Can you work these out from the model? Positions are in its coordinate system, mm. A direction names the side the tool comes from. Give positions to 0.01 mm unless a question says otherwise; leave off trailing zeros. Loops run counter-clockwise (first coordinate to the right, second up) from the corner with the lowest first, then second, coordinate; pieces in that order, holes last. Notation, with made-up numbers: M -36.5,-35 L 1.5,-35 A23 cw 1.5,-15 Z; hole C 9.5,0 d7. An arc over 180 degrees is marked long. Answer as a JSON object with one key per item and string values.
```python
from build123d import *

# Parameters (mm, degrees)
SKETCH1_W                = 32
SKETCH1_H                = 15
BOSS_EXTRUDE1_DEPTH      = 4
BOSS_EXTRUDE2_START      = 4
SKETCH1_3_W              = 32
SKETCH1_3_H              = 5
BOSS_EXTRUDE2_DEPTH      = 23.5
BOSS_EXTRUDE3_DEPTH      = 17
M3_CLEARANCE_HOLE1_D     = 3.6
M3_CLEARANCE_HOLE1_DEPTH = 10
M3_CLEARANCE_HOLE1_TIP   = 1.081549114


with BuildPart() as part:
    # Sketch1 → Boss-Extrude1 (new body)
    with BuildSketch(Plane(origin=(0, 0, 0), x_dir=(1, 0, 0), z_dir=(0, 1, 0))):
        with Locations((0, 2.5)):
            Rectangle(SKETCH1_W, SKETCH1_H)
    extrude(amount=BOSS_EXTRUDE1_DEPTH)

    # Sketch1<3> → Boss-Extrude2 (add)
    with BuildSketch(Plane(origin=(0, 0, 0), x_dir=(1, 0, 0), z_dir=(0, 1, 0)).offset(BOSS_EXTRUDE2_START)):
        with Locations((0, -2.5)):
            Rectangle(SKETCH1_3_W, SKETCH1_3_H)
    extrude(amount=BOSS_EXTRUDE2_DEPTH)

    # Sketch2 → Boss-Extrude3 (add)
    with BuildSketch(Plane.XY.offset(5)):
        Polygon((-6.5, 2), (-6.5, 25.5), (-2.5, 25.5), (-2.5, 27.5), (-9, 27.5), (-9, 0), (9, 0), (9, 27.5), (2.5, 27.5), (2.5, 25.5), (6.5, 25.5), (6.5, 2), align=None)
    extrude(amount=BOSS_EXTRUDE3_DEPTH)

    # M3 Clearance Hole1
    with Locations(Plane(origin=(0, 4, 0), x_dir=(1, 0, 0), z_dir=(0, 1, 0))):
        with Locations((-10, 5), (10, 5)):
            Hole(M3_CLEARANCE_HOLE1_D / 2, depth=M3_CLEARANCE_HOLE1_DEPTH)
            with Locations((0, 0, -(M3_CLEARANCE_HOLE1_DEPTH + M3_CLEARANCE_HOLE1_TIP / 2))):  # 118° drill point
                Cone(0, M3_CLEARANCE_HOLE1_D / 2, M3_CLEARANCE_HOLE1_TIP, mode=Mode.SUBTRACT)


solid = part.part
```
1) Suppose I cut it at D-D, the plane z = 12. Write out the boundary of the cut face in (x, y), and give its area (4 significant figures).
Answer list:
{"outline": "M -9,0 L 9,0 L 9,27.5 L 2.5,27.5 L 2.5,25.5 L 6.5,25.5 L 6.5,2 L -6.5,2 L -6.5,25.5 L -2.5,25.5 L -2.5,27.5 L -9,27.5 Z", "area": "179.5 mm^2"}
2) Please list where these lines run through material, in increasing order: line 1 along X through (y, z) = (1.25, -5); line 2 along X through (y, z) = (15.75, 8); line 3 along Z through (x, y) = (10, 0.8). Write a range as from..to.
Answer list:
{"line 1": "-16..-11.8, -8.2..8.2, 11.8..16", "line 2": "-9..-6.5, 6.5..9", "line 3": "-10..-6.8, -3.2..5"}
3) Suppose I cut it at C-C, the plane y = 23. Write out the boundary of the cut face in (x, z), and give its area (3 significant figures).
Answer list:
{"outline": "M -16,0 L 16,0 L 16,5 L 9,5 L 9,22 L 6.5,22 L 6.5,5 L -6.5,5 L -6.5,22 L -9,22 L -9,5 L -16,5 Z", "area": "245 mm^2"}
4) Will these pins go through, and if not, where does the flat tip stop? pin 1 Ø12 at (x, y) = (-6, 16) entering from +Z; pin 2 Ø5 at (y, z) = (7, 15.5) entering from -X; pin 3 Ø12 at (x, y) = (-3.5, 16.5) entering from -Z; pin 4 Ø13.5 at (y, z) = (10, 15.5) entering from +X.
Answer list:
{"pin 1": "z = 22", "pin 2": "x = -9", "pin 3": "z = 0", "pin 4": "x = 9"}
5) If we mould it in two halves opening along Z, with no side actions, what happens to faces 5 (the flat face through (-5, 25.5, 13)), 6 (the flat face through (12, 14, 5)), 7 (the cylindrical face through (-8.572, 1.972, -3.905)), 8 (the cylindrical face through (11.428, 1.972, -3.905))? For each: +Z half, -Z half, draft (parallel to the pull), parting line (faces both ways), or undercut.
Answer list:
{"face 5": "draft", "face 6": "+Z half", "face 7": "undercut", "face 8": "undercut"}
6) Suppose I cut it at B-B, the plane z = -5. Write out the boundary of the cut face in (x, y), and give its area (3 significant figures).
Answer list:
{"outline": "M -16,0 L -11.8,0 L -11.8,4 L -16,4 Z; M -8.2,0 L 8.2,0 L 8.2,4 L -8.2,4 Z; M 11.8,0 L 16,0 L 16,4 L 11.8,4 Z", "area": "99.2 mm^2"}
7) For faces 1 (the flat face through (4, 25.5, 13)), 2 (the flat face through (-9, 14, 13)), 3 (the flat face through (-2.5, 26, 13)), 4 (the flat face through (0, 16, 0)), which set-ups out of +Z, -Z, +X, -X, +Y, -Y let a thin tool reach every point of the face, with its end or its side?
Answer list:
{"face 1": "+Z", "face 2": "+Z, -X, +Y, -Y", "face 3": "+Z, +Y", "face 4": "-Z, +X, -X, +Y"}
8) Suppose I cut it at A-A, the plane x = -10. Write out the boundary of the cut face in (y, z), and give its area (3 significant figures).
Answer list:
{"outline": "M 0,-10 L 4,-10 L 4,-6.8 L 0,-6.8 Z; M 0,-3.2 L 4,-3.2 L 4,0 L 27.5,0 L 27.5,5 L 0,5 Z", "area": "163 mm^2"}
